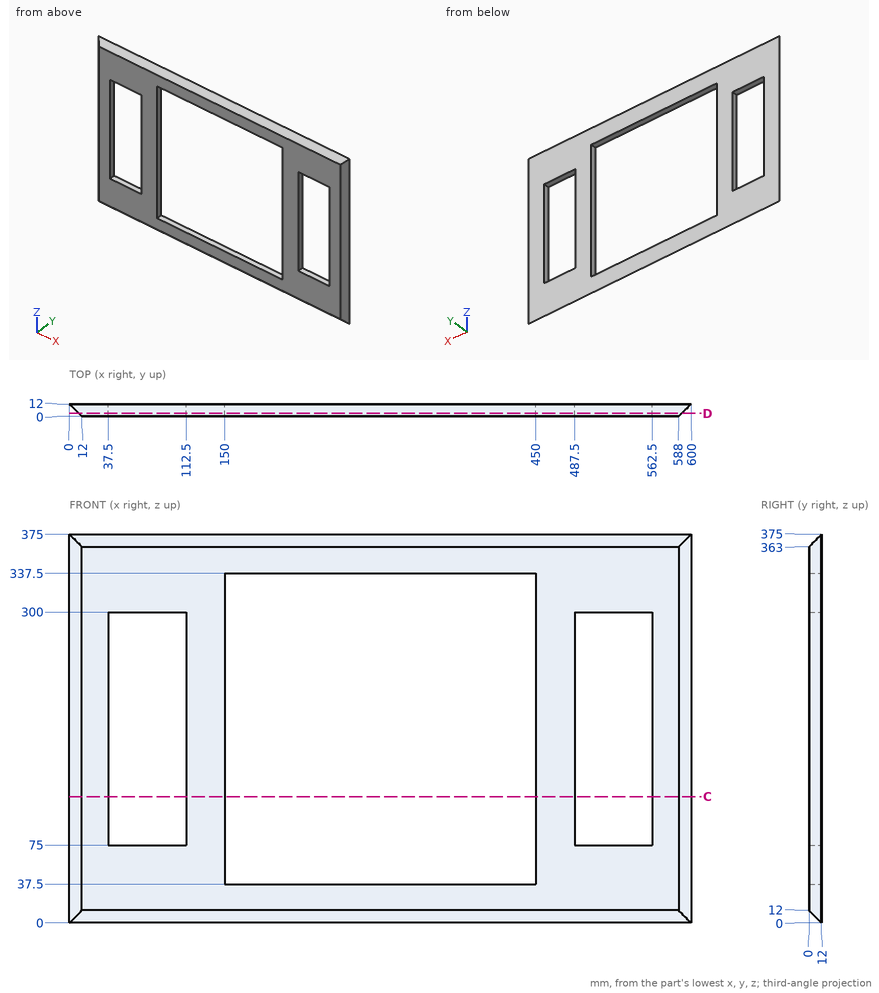
Design review of the part shown in the three views and the two pictorial views. Dimensions are in mm from the part's minimum x, y and z. Coordinates: 2 decimals unless noted, no trailing zeros. Order: outer loops, then holes, each group sorted by start corner. A loop starts at its lowest first (then second) coordinate and runs counter-clockwise, first axis right, second up.
1) Take a section at D-D, the plane y = 3. Give the boundary of the cut face in (x, z).
2) Wall thickness on line 1 along X through (y, z) = (9, 231.5); line 2 along X through (y, z) = (1.75, 221); line 3 along Z through (x, y) = (414, 6): over which ranges is each line inside the solid? List them lowest first.
3) Clearance check with flat-ended pins moving along their axes: pin 1 (6 mm diameter, centred on y = 4.5, z = 225.5, fed in from -X); pin 2 (3 mm diameter, centred on x = 288.5, y = 3.5, fed in from +Z); pin 3 (6 mm diameter, centred on x = 89.5, y = 6.5, fed in from -Z). State where each tip first meets the part, or that it passes through.
4) Take a section at C-C, the plane z = 122. State how many separate pieces and enclosed holes the cut face has, and give its area (3 significant figures).
Returned:
1. outline: (9, 9) - (591, 9) - (591, 366) - (9, 366) - close; hole (37.5, 75) - (112.5, 75) - (112.5, 300) - (37.5, 300) - close; hole (150, 37.5) - (450, 37.5) - (450, 337.5) - (150, 337.5) - close; hole (487.5, 75) - (562.5, 75) - (562.5, 300) - (487.5, 300) - close
2. line 1: x = 3 to 37.5, 112.5 to 150, 450 to 487.5, 562.5 to 597
2. line 2: x = 10.25 to 37.5, 112.5 to 150, 450 to 487.5, 562.5 to 589.75
2. line 3: z = 6 to 37.5, 337.5 to 369
3. pin 1: stops at x = 4.5
3. pin 2: stops at z = 368
3. pin 3: stops at z = 2.5
4. separate pieces: 4
4. enclosed holes: 0
4. area: 1,660 mm2
